For this review, take the finished solid that the model builds, in its own axes (mm). Round coordinates to 2 decimals unless told otherwise and drop trailing zeros. Write each loop counter-clockwise with the first axis right and the second up, starting at its lowest first coordinate (ties: lowest second). Pieces come first, ordered by that corner, then holes.
Autodesk Inventor part; units mm, degrees
ref_plane "YZ Plane" through (0, 0, 0) normal (1, 0, 0) x (0, 1, 0)
ref_plane "XZ Plane" through (0, 0, 0) normal (0, 1, 0) x (-1, 0, 0)
ref_plane "XY Plane" through (0, 0, 0) normal (0, 0, 1) x (1, 0, 0)
sketch "Sketch1" plane through (0, 0, 0) normal (0, 0, 1) x (1, 0, 0)
  line L0 (0, 0) -> (0, 15)
  line L1 (0, 15) -> (-15, 15)
  line L2 (-15, 0) -> (-15, 15)
  line L3 (0, 0) -> (-15, 0)
  line L4 (-15, 15) -> (-515, 15)
  line L5 (-15, 0) -> (-515, 0)
  line L6 (-15, -360) -> (-15, 0)
  line L7 (0, -360) -> (0, 0)
  line L8 (-115, -360) -> (-115, 0)
  line L9 (-130, -360) -> (-130, 0)
  line L10 (-128, 13) -> (-2, 13)
  line L11 (-2, 13) -> (-2, -37)
  line L12 (-2, -37) -> (-128, -37)
  line L13 (-128, -37) -> (-128, 13)
  line L14 (-13, 13) -> (-13, 2)
  line L15 (-13, 2) -> (-2, 2)
extrude "Extrusion1" add sketch "Sketch1" along normal blind 4 contours L11 L12 L6 L3 | L3 L2 L10 L14 L15 L11 | L5 L13 L10 L2 | L6 L12 L8 L5 | L8 L12 L13 L5
sketch "Sketch2" plane through (0, 0, 4) normal (0, 0, 1) x (1, 0, 0)
  line L0 (-13, 13) -> (-128, 13)
  line L1 (-128, 13) -> (-128, -37)
  line L2 (-128, -37) -> (-2, -37)
  line L3 (-2, -37) -> (-2, 2)
  line L4 (-13, 2) -> (-13, 13)
  line L5 (-2, 2) -> (-13, 2)
  point P0 (0, 0)
  point P1 (-122.5, -32.4606)
  point P2 (-122.5, 7.5)
  point P3 (-25, 7.5)
  point P4 (-7.5, -32.4606)
  dimension "d6" = 5.5
  dimension "d7" = 5.5
  dimension "d8" = 5.5
  dimension "d9" = 23
hole "Hole1" at (-122.5, -32.4606, 4) at (-122.5, 7.5, 4) at (-25, 7.5, 4) at (-7.5, -32.4606, 4) direction (0, 0, -1) diameter 3.7 depth 8 tip angle 118
fillet "Fillet1" radius 5 6 edges at (-2, -37, 2) (-128, -37, 2) (-128, 13, 2) (-13, 13, 2) (-13, 2, 2) (-2, 2, 2)
equation "\"d1\" = d0"
equation "\"d3\" = d1"
equation "\"d21\" = d20"
properties part number "Frame_Foot_Solid" material "ABS Plastic"
(1) For line 1 along Y through (x, z) = (-122.5, 1.2); line 2 along X through (y, z) = (7.5, 1.85); line 3 along Y through (x, z) = (-25, 3), list the stretches that pass through material, from the lowest coordinate up.
Geometry check:
line 1: y = -37 to -34.31, -30.61 to 5.65, 9.35 to 13
line 2: x = -128 to -124.35, -120.65 to -26.85, -23.15 to -13
line 3: y = -37 to 5.65, 9.35 to 13
(2) We need section A-A, the plane x = -25. Give the boundary of the cut face in (y, z), and give its area (3 significant figures).
Geometry check:
outline: (-37, 0) - (5.65, 0) - (5.65, 4) - (-37, 4) - close; (9.35, 0) - (13, 0) - (13, 4) - (9.35, 4) - close
area: 185 mm2
(3) For pin 1 Ø3.5 at (x, y) = (-122.5, 7.5) entering from -Z; pin 2 Ø1.1 at (y, z) = (7.5, 2.5) entering from +X; pin 3 Ø1.1 at (x, z) = (-7.5, 1.5) entering from +Y, all flat-tipped, find the tip position at first contact; note any pin that passes through.
Geometry check:
pin 1: passes through
pin 2: stops at x = -13
pin 3: stops at y = 2
(4) We need section B-B, the plane z = 3.3. Give the boundary of the cut face in (x, y).
Geometry check:
outline: (-128, -32) arc R5 ccw to (-123, -37) - (-7, -37) arc R5 ccw to (-2, -32) - (-2, -3) arc R5 ccw to (-7, 2) - (-8, 2) arc R5 cw to (-13, 7) - (-13, 8) arc R5 ccw to (-18, 13) - (-123, 13) arc R5 ccw to (-128, 8) - close; hole circle Ø3.7 at (-122.5, -32.46); hole circle Ø3.7 at (-122.5, 7.5); hole circle Ø3.7 at (-25, 7.5); hole circle Ø3.7 at (-7.5, -32.46)
(5) Mouldability with a two-part tool opening along Y and no side actions: class faces 1 (the face through (-4, -36, 2)), 2 (the face through (-124.334, -32.22, 1.972)), 3 (the face through (-12, 4, 2)), 4 (the face through (-124.334, 7.741, 1.972)) as pulls with the +Y half, pulls with the -Y half, needs draft (parallel to the pull), parting line crosses it, or undercut.
Geometry check:
face 1: pulls with the -Y half
face 2: undercut
face 3: pulls with the +Y half
face 4: undercut
